```python
from build123d import *

# Parameters (mm, degrees)
F0_R     = 6.35
F1_DEPTH = 41.275
F2_R     = 4.953
F3_DEPTH = 38.1
F5_R     = 3.7719
F6_DEPTH = 3.175
F7_R     = 1.905


with BuildPart() as f1:
    # F0 (on Top) → F1 (new body)
    with BuildSketch(Plane.XY):
        Circle(F0_R)
    extrude(amount=F1_DEPTH)

    # F2 (on Top) → F3 (cut)
    with BuildSketch(Plane.XY):
        Circle(F2_R)
    extrude(amount=F3_DEPTH, mode=Mode.SUBTRACT)

    # F5 (on offset) → F6 (cut, through all)
    with BuildSketch(Plane.XY.offset(41.275)):
        Circle(F5_R)
    extrude(amount=-F6_DEPTH, mode=Mode.SUBTRACT)

    # F7
    f7_edges = [f1.edges().sort_by_distance(p)[0] for p in [
        (-6.35, 0, 41.275),
    ]]
    fillet(f7_edges, radius=F7_R)


solid = f1.part
```
The listing builds one solid part. Answer for the finished solid, in the listing's coordinates (mm). A direction names the side the tool comes from. Coordinates: 2 decimals unless noted, no trailing zeros. Write each loop counter-clockwise with the first axis right and the second up, starting at its lowest first coordinate (ties: lowest second). Pieces come first, ordered by that corner, then holes.
Q1. Find the intervals of material crossed by line 1 along Y through (x, z) = (0, 11); line 2 along Y through (x, z) = (0, 38.85), in increasing order.
Returned:
line 1: y = -6.35 to -4.95, 4.95 to 6.35
line 2: y = -6.35 to -3.77, 3.77 to 6.35
Q2. The mould has two halves that part along X. Classify faces 1 (the cylindrical face through (-1.38, -6.2, 19.41)), 2 (the flat face through (-1, -4, 41.275)), 3 (the cylindrical face through (-0.64, 4.91, 18.78)): released by +X, released by -X, zero draft, split by the parting line, or undercut.
Returned:
face 1: split by the parting line
face 2: zero draft
face 3: undercut
Q3. Which of the six approach directions +Z, -Z, +X, -X, +Y, -Y give full straight-line access (tool end or side, diameter ignored) to faces 4 (the cylindrical face through (-2.99, -2.3, 39.71)), 5 (the flat face through (-1, -4, 38.1))?
Returned:
face 4: +Z, -Z
face 5: -Z
Q4. Section A-A, the plane x = 0 is taken. Write down the section's boundary in (y, z) (3 decimals).
Returned:
outline: (-6.35, 0) - (-4.953, 0) - (-4.953, 38.1) - (-3.772, 38.1) - (-3.772, 41.275) - (-4.445, 41.275) arc R1.905 ccw to (-6.35, 39.37) - close; (3.772, 38.1) - (4.953, 38.1) - (4.953, 0) - (6.35, 0) - (6.35, 39.37) arc R1.905 ccw to (4.445, 41.275) - (3.772, 41.275) - close
Q5. Given P1, Ø7, axis at x = 0, y = 0, coming from the +Z side; P2, Ø6, axis at y = -5, z = 13.5, coming from the -X side; P3, Ø1, axis at x = -5, z = 26, coming from the +Y side; P4, Ø6, axis at x = -2, z = 7, coming from the -Y side, each flat-ended and moving along its own axis, determine where each tip first touches the part or whether it passes through.
Returned:
P1: passes through
P2: stops at x = -6.03
P3: stops at y = 4.48
P4: stops at y = -6.35
Q6. Section C-C, the plane z = 15.5 is taken. Write down the section's boundary in (x, y), then the cut area to 3 significant figures.
Returned:
outline: circle Ø12.7 at (0, 0); hole circle Ø9.91 at (0, 0)
area: 49.6 mm2
